from build123d import *

# Parameters (mm, degrees)
SKETCH1_W           = 31.5
SKETCH1_H           = 31.5
BOSS_EXTRUDE1_DEPTH = 22
FILLET2_R           = 2
SKETCH2_R           = 15.164213562
BOSS_EXTRUDE2_DEPTH = 0.3
SKETCH3_R           = 14
BOSS_EXTRUDE3_DEPTH = 0.3
SKETCH4_R           = 13
SKETCH4_R_2         = 11
BOSS_EXTRUDE5_DEPTH = 4
SKETCH6_R           = 11
BOSS_EXTRUDE6_DEPTH = 8
BOSS_EXTRUDE6_TAPER = 50


with BuildPart() as part:
    # Sketch1 → Boss-Extrude1 (new body)
    with BuildSketch(Plane.XY):
        with Locations((15.75, 15.75)):
            Rectangle(SKETCH1_W, SKETCH1_H)
    extrude(amount=BOSS_EXTRUDE1_DEPTH)

    # Fillet2
    fillet2_edges = [part.edges().sort_by_distance(p)[0] for p in [
        (0, 0, 11),
        (0, 31.5, 11),
        (31.5, 31.5, 11),
        (31.5, 0, 11),
    ]]
    fillet(fillet2_edges, radius=FILLET2_R)

    # Sketch2 → Boss-Extrude2 (add)
    with BuildSketch(Plane.XY.offset(22)):
        with Locations((15.75, 15.75)):
            Circle(SKETCH2_R)
    extrude(amount=BOSS_EXTRUDE2_DEPTH)

    # Sketch3 → Boss-Extrude3 (add)
    with BuildSketch(Plane.XY.offset(22.3)):
        with Locations((15.75, 15.75)):
            Circle(SKETCH3_R)
    extrude(amount=BOSS_EXTRUDE3_DEPTH)

    # Sketch4 → Boss-Extrude5 (add)
    with BuildSketch(Plane.XY.offset(22.6)):
        with Locations((15.75, 15.75)):
            Circle(SKETCH4_R)
        with Locations((15.75, 15.75)):
            Circle(SKETCH4_R_2, mode=Mode.SUBTRACT)
    extrude(amount=BOSS_EXTRUDE5_DEPTH)

    # Sketch6 → Boss-Extrude6 (add)
    with BuildSketch(Plane.XY.offset(22.6)):
        with Locations((15.75, 15.75)):
            Circle(SKETCH6_R)
    extrude(amount=BOSS_EXTRUDE6_DEPTH, taper=BOSS_EXTRUDE6_TAPER)


solid = part.part
Design review of the part built by this model. Coordinates are the model's own, in mm. A direction names the side the tool comes from. Give positions to 0.01 mm unless a question says otherwise; leave off trailing zeros. Write each loop counter-clockwise with the first axis right and the second up, starting at its lowest first coordinate (ties: lowest second). Pieces come first, ordered by that corner, then holes. Notation, with made-up numbers: M -31,-26.75 L 13,-26.75 A4 ccw 13,-19.75 Z; hole C -32.5,41 d7. An arc over 180 degrees is marked long. Return JSON: item names as keys, results as strings. Group by question number.
Item 1: The part is to be moulded in two halves that separate along Y. For faces 3 (the cylindrical face through (0.57, 30.9, 11.15)), 4 (the conical face through (13.379, 13.932, 29.323)), 5 (the cylindrical face through (30.9, 0.57, 11.15)), 6 (the flat face through (20, 3, 22.6)), say which applies: pulls with the +Y half, pulls with the -Y half, needs draft (parallel to the pull), parting line crosses it, or undercut.
Item 2: Wall thickness on line 1 along Y through (x, z) = (15.75, 24.85); line 2 along Y through (x, z) = (15.75, 23.5); line 3 along X through (y, z) = (15, 24): over which ranges is each line inside the solid? List them lowest first.
Item 3: Take a section at D-D (y = 4). Give the boundary of the cut face in (x, z).
Item 4: Clearance check with flat-ended pins moving along their axes: pin 1 Ø5 at (x, y) = (24, 14) entering from -Z; pin 2 Ø6 at (x, z) = (23, 26) entering from -Y; pin 3 Ø16 at (x, y) = (22.5, 9) entering from +Z. State where each tip first meets the part, or that it passes through.
Item 5: Take a section at C-C (z = 28). Give the boundary of the cut face in (x, y).
Item 6: Take a section at A-A (y = 15.75). Give the boundary of the cut face in (x, z), plus the area to 3 significant figures.
Item 7: Tool access review of faces 1 (the flat face through (16, 0, 11)), 2 (the flat face through (29.2, 11.3, 22.3)): name each direction out of +Z, -Z, +X, -X, +Y, -Y from which nothing blocks a thin tool from reaching the whole face with its end or side.
Return value:
{
 "1": {"face 3": "pulls with the +Y half", "face 4": "undercut", "face 5": "pulls with the -Y half", "face 6": "needs draft"},
 "2": {"line 1": "y = 2.75 to 4.75, 7.43 to 24.07, 26.75 to 28.75", "line 2": "y = 2.75 to 4.75, 5.82 to 25.68, 26.75 to 28.75", "line 3": "x = 2.77 to 4.78, 6.45 to 25.05, 26.72 to 28.73"},
 "3": {"outline": "M 0,0 L 31.5,0 L 31.5,22 L 25.34,22 L 25.34,22.3 L 23.36,22.3 L 23.36,22.6 L 21.31,22.6 L 21.31,26.6 L 10.19,26.6 L 10.19,22.6 L 8.14,22.6 L 8.14,22.3 L 6.16,22.3 L 6.16,22 L 0,22 Z"},
 "4": {"pin 1": "stops at z = 0", "pin 2": "stops at y = 3.46", "pin 3": "stops at z = 30.53"},
 "5": {"outline": "C 15.75,15.75 d9.13"},
 "6": {"outline": "M 0,0 L 31.5,0 L 31.5,22 L 30.91,22 L 30.91,22.3 L 29.75,22.3 L 29.75,22.6 L 28.75,22.6 L 28.75,26.6 L 26.75,26.6 L 26.75,22.6 L 17.22,30.6 L 14.28,30.6 L 4.75,22.6 L 4.75,26.6 L 2.75,26.6 L 2.75,22.6 L 1.75,22.6 L 1.75,22.3 L 0.59,22.3 L 0.59,22 L 0,22 Z", "area": "826 mm2"},
 "7": {"face 1": "+Z, -Z, +X, -X, -Y", "face 2": "+Z"}
}
